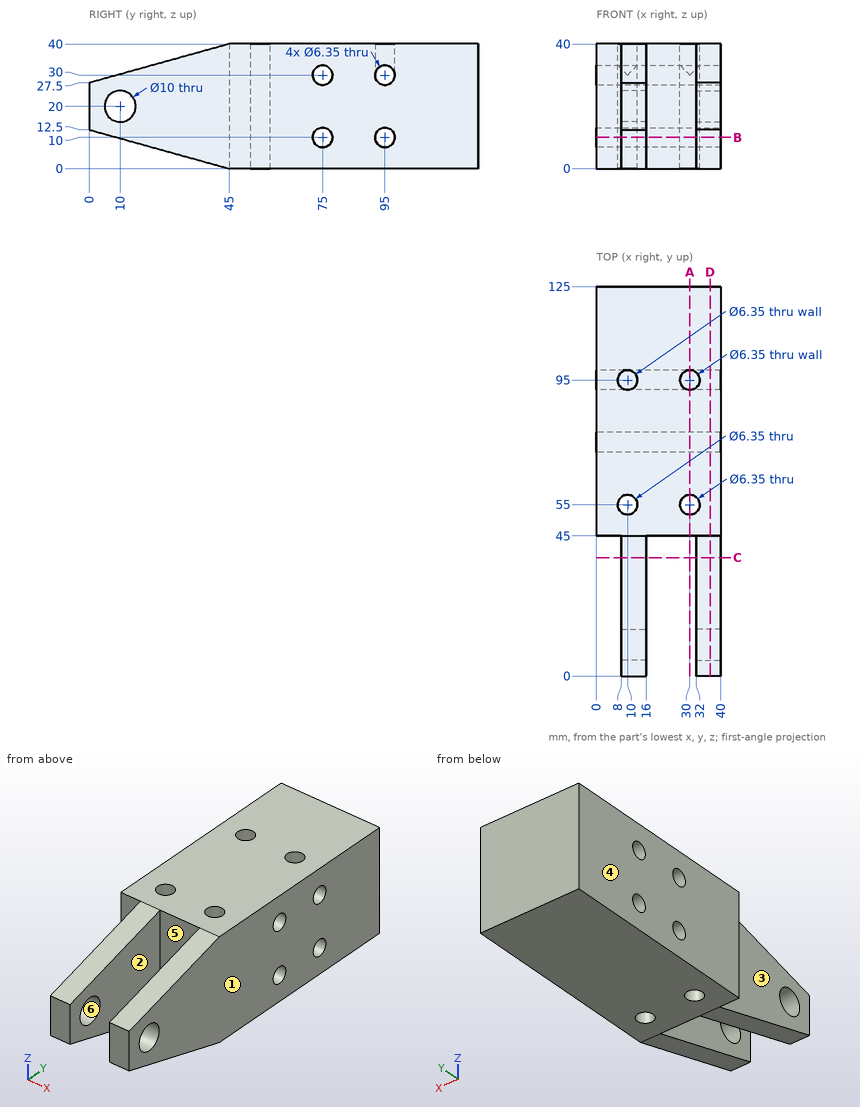
Verification items for this drawing (mm, ordinates from the low corner). A direction names the side the tool comes from. Round coordinates to 2 decimals unless told otherwise and drop trailing zeros. Write each loop counter-clockwise with the first axis right and the second up, starting at its lowest first coordinate (ties: lowest second). Pieces come first, ordered by that corner, then holes. Notation, with made-up numbers: (-8, -34.75) - (11, -34.75) arc R20 ccw to (11, -16.75) - close; hole circle Ø10 at (35.5, 18.5). An arc over 180 degrees is marked (long way). Answer as a JSON object with one key per item and string values. Group by question number.
Q1. Section check D-D, the plane x = 36.5. Enter the section's corners in (y, z) (3 decimals).
Q2. Section check A-A, the plane x = 30. Enter the section's corners in (y, z) (3 decimals).
Q3. Section check C-C, the plane y = 38. Enter the section's corners in (x, z), plus the area to 3 significant figures.
Q4. Go/stop test with flat-tipped pins: pin 1 Ø12 at (y, z) = (19, 16) entering from -X; pin 2 Ø8 at (x, z) = (24, 12.5) entering from -Y. Record where each tip stops, or that it passes through.
Q5. Tool access check on the marked faces 1, 2 and 3. Record the directions out of +Z, -Z, +X, -X, +Y, -Y that give a thin tool (end or side, any length) a straight path to the whole face; none if there is none.
Q6. Thickness scan on line 1 (Z direction, x = 35.5, y = 95) (3 decimals); line 2 (X direction, y = 44.5, z = 11.5). Record the ranges inside material, lowest first.
Q7. Mould release check, pull along Y, two halves, no side actions. Record for the marked faces 4, 5 and 6: released by +Y, released by -Y, zero draft, split by the parting line, or undercut.
Q8. Section check B-B, the plane z = 10. Enter the section's corners in (x, y) (3 decimals), plus the area to 3 significant figures.
Found:
{
 "1": {"outline": "(0, 12.5) - (45, 0) - (125, 0) - (125, 40) - (45, 40) - (0, 27.5) - close; hole circle Ø10 at (10, 20); hole circle Ø6.35 at (75, 10); hole circle Ø6.35 at (75, 30); hole circle Ø6.35 at (95, 10); hole circle Ø6.35 at (95, 30)"},
 "2": {"outline": "(45, 0) - (51.825, 0) - (51.825, 40) - (45, 40) - close; (58.175, 0) - (125, 0) - (125, 40) - (98.175, 40) - (98.175, 30) arc R3.175 cw to (91.825, 30) - (91.825, 40) - (58.175, 40) - close; hole circle Ø6.35 at (75, 10); hole circle Ø6.35 at (75, 30); hole circle Ø6.35 at (95, 10)"},
 "3": {"outline": "(8, 1.94) - (16, 1.94) - (16, 38.06) - (8, 38.06) - close; (32, 1.94) - (40, 1.94) - (40, 38.06) - (32, 38.06) - close", "area": "578 mm^2"},
 "4": {"pin 1": "stops at x = 8", "pin 2": "stops at y = 45"},
 "5": {"face 1": "+Z, -Z, +X, +Y, -Y", "face 2": "+Z, -Z, -Y", "face 3": "+Z, -Z, -X, -Y"},
 "6": {"line 1": "z = 0 to 6.825, 13.175 to 26.825, 33.175 to 40", "line 2": "x = 8 to 16, 32 to 40"},
 "7": {"face 4": "zero draft", "face 5": "released by -Y", "face 6": "undercut"},
 "8": {"outline": "(0, 45) - (8, 45) - (8, 9) - (16, 9) - (16, 45) - (32, 45) - (32, 9) - (40, 9) - (40, 71.825) - (0, 71.825) - close; (0, 78.175) - (40, 78.175) - (40, 91.825) - (0, 91.825) - close; (0, 98.175) - (40, 98.175) - (40, 125) - (0, 125) - close; hole circle Ø6.35 at (10, 55); hole circle Ø6.35 at (30, 55)", "area": "3,200 mm^2"}
}
